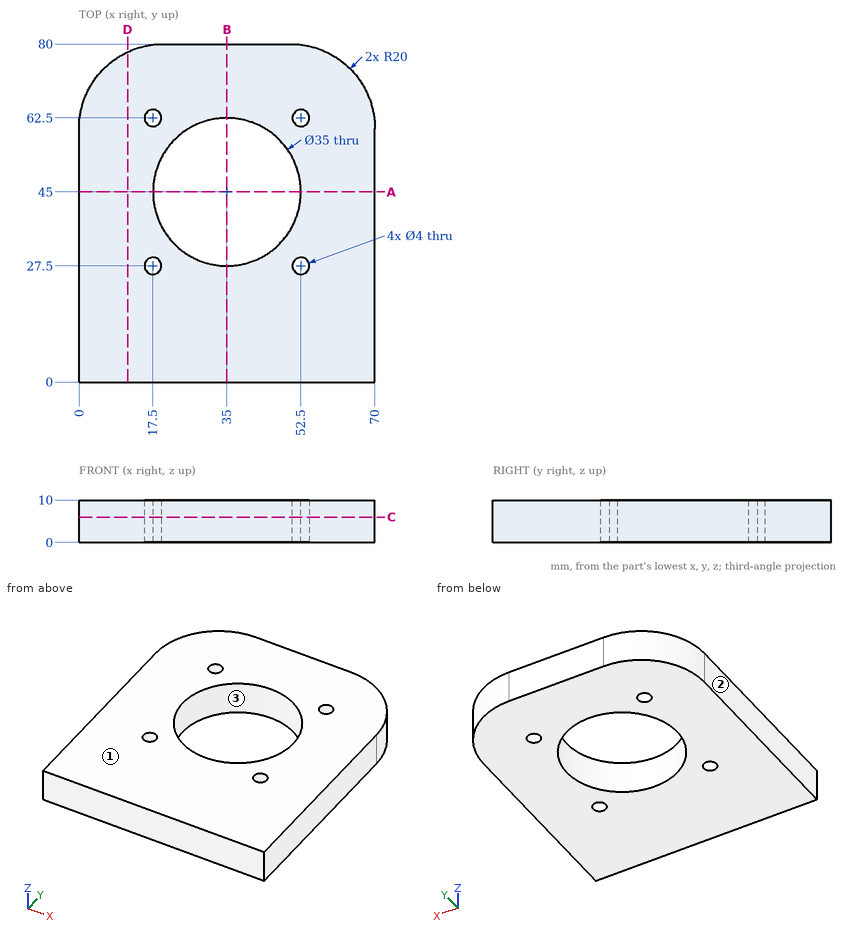
Here's the drawing with two shaded views (mm, measured from the low corner). I have some questions. Give positions to 0.01 mm unless a question says otherwise; leave off trailing zeros. Order: outer loops, then holes, each group sorted by start corner. A loop starts at its lowest first (then second) coordinate and runs counter-clockwise, first axis right, second up. Notation, with made-up numbers: M 76,-34 L 91,-34 A31 cw 91,-4 Z; hole C 30,39 d8. An arc over 180 degrees is marked long. One line per question, with ' | ' between items.
Item 1: Suppose I cut it at A-A, the plane y = 45. Write out the boundary of the cut face in (x, z), then the cut area to 3 significant figures.
Answer block:
outline: M 0,0 L 17.5,0 L 17.5,10 L 0,10 Z; M 52.5,0 L 70,0 L 70,10 L 52.5,10 Z | area: 350 mm2
Item 2: Suppose I cut it at D-D, the plane x = 11.5. Write out the boundary of the cut face in (y, z), then the cut area to 3 significant figures.
Answer block:
outline: M 0,0 L 78.1,0 L 78.1,10 L 0,10 Z | area: 781 mm2
Item 3: We'd pull the mould along X, two halves only. Please class the marked faces 1, 2 and 3: released by +X, released by -X, zero draft, split by the parting line, or undercut.
Answer block:
face 1: zero draft | face 2: released by -X | face 3: undercut
Item 4: Suppose I cut it at C-C, the plane z = 6. Write out the boundary of the cut face in (x, y), then the cut area to 3 significant figures.
Answer block:
outline: M 0,0 L 70,0 L 70,60 A20 ccw 50,80 L 20,80 A20 ccw 0,60 Z; hole C 17.5,27.5 d4; hole C 17.5,62.5 d4; hole C 35,45 d35; hole C 52.5,27.5 d4; hole C 52.5,62.5 d4 | area: 4,420 mm2
Item 5: Suppose I cut it at B-B, the plane x = 35. Write out the boundary of the cut face in (y, z).
Answer block:
outline: M 0,0 L 27.5,0 L 27.5,10 L 0,10 Z; M 62.5,0 L 80,0 L 80,10 L 62.5,10 Z
Item 6: Please list where these lines run through material, in increasing order: L1, parallel to Y at x = 35, z = 4; L2, parallel to X at y = 64, z = 8.5; L3, parallel to X at y = 53.5, z = 5.25.
Answer block:
L1: y = 0 to 27.5, 62.5 to 80 | L2: x = 0.4 to 16.18, 18.82 to 51.18, 53.82 to 69.6 | L3: x = 0 to 19.7, 50.3 to 70
